from build123d import *

# Parameters (mm, degrees)
F1_DEPTH = 381
F3_DEPTH = 50.8


with BuildPart() as f1:
    # F0 (on Front) → F1 (new body, symmetric)
    with BuildSketch(Plane.XZ):
        with BuildLine():
            ThreePointArc((38.1, 25.4), (34.3802561211, 34.3802561211), (25.4, 38.1))
            Line((25.4, 38.1), (-25.4, 38.1))
            ThreePointArc((-25.4, 38.1), (-34.3802561211, 34.3802561211), (-38.1, 25.4))
            Line((-38.1, 25.4), (-38.1, -25.4))
            ThreePointArc((-38.1, -25.4), (-34.3802561211, -34.3802561211), (-25.4, -38.1))
            Line((-25.4, -38.1), (25.4, -38.1))
            ThreePointArc((25.4, -38.1), (34.3802561211, -34.3802561211), (38.1, -25.4))
            Line((38.1, -25.4), (38.1, 25.4))
        make_face()
        with BuildLine():
            ThreePointArc((25.4, 31.7500010133), (29.890128777, 29.890128777), (31.7500010133, 25.4))
            Line((31.7500010133, 25.4), (31.7500010133, -25.4))
            ThreePointArc((31.7500010133, -25.4), (29.890128777, -29.890128777), (25.4, -31.7500010133))
            Line((25.4, -31.7500010133), (-25.4, -31.7500010133))
            ThreePointArc((-25.4, -31.7500010133), (-29.890128777, -29.890128777), (-31.7500010133, -25.4))
            Line((-31.7500010133, -25.4), (-31.7500010133, 25.4))
            ThreePointArc((-31.7500010133, 25.4), (-29.890128777, 29.890128777), (-25.4, 31.7500010133))
            Line((-25.4, 31.7500010133), (25.4, 31.7500010133))
        make_face(mode=Mode.SUBTRACT)
    extrude(amount=F1_DEPTH, both=True)

    # F2 (on Top) → F3 (cut, symmetric)
    with BuildSketch(Plane.XY):
        Polygon((38.1, -304.8), (-38.1, -381), (38.1, -381), align=None)
        Polygon((38.1, 381), (-38.1, 381), (38.1, 304.8), align=None)
    extrude(amount=F3_DEPTH, both=True, mode=Mode.SUBTRACT)


solid = f1.part
Work out the finished part from the listing and answer in its coordinate system (mm). A direction names the side the tool comes from. Give positions to 0.01 mm unless a question says otherwise; leave off trailing zeros. Write each loop counter-clockwise with the first axis right and the second up, starting at its lowest first coordinate (ties: lowest second). Pieces come first, ordered by that corner, then holes. Notation, with made-up numbers: (43.5, -2.75) - (76.5, -2.75) arc R35 cw to (76.5, 34.25) - close; hole circle Ø4 at (-30.5, 64.25). An arc over 180 degrees is marked (long way). One line per item, written item: value. Start each with the question number.
1. For a pull along Z with two mould halves and no side action, classify faces 3 (the cylindrical face through (34.48, -4.44, 34.28)), 4 (the cylindrical face through (34.28, -4.44, -34.48)), 5 (the flat face through (31.75, -4, 0)) as +Z half, -Z half, draft (parallel to the pull), parting line (faces both ways), or undercut.
2. Find section C-C (y = -79.5). Write down the section's boundary in (x, z), then the cut area to 3 significant figures.
3. Consider probe 1 along Z at (x, y) = (-1, -38.5); probe 2 along Z at (x, y) = (28, 147). Determine where each line is inside the solid, lowest interval first.
4. For faces 1 (the flat face through (-31.75, -5, 0)), 2 (the cylindrical face through (-34.48, -5.33, -34.28)), determine the directions among +Z, -Z, +X, -X, +Y, -Y from which every point of the face is accessible in a straight line to the end or side of a thin tool.
5. Find section A-A (x = -19). Write down the section's boundary in (y, z), then the cut area to 3 significant figures.
6. Find section B-B (z = 2.5). Write down the section's boundary in (x, y).
Geometry results:
1. face 3: +Z half
1. face 4: -Z half
1. face 5: undercut
2. outline: (-38.1, -25.4) arc R12.7 ccw to (-25.4, -38.1) - (25.4, -38.1) arc R12.7 ccw to (38.1, -25.4) - (38.1, 25.4) arc R12.7 ccw to (25.4, 38.1) - (-25.4, 38.1) arc R12.7 ccw to (-38.1, 25.4) - close; hole (-31.75, -25.4) arc R6.35 ccw to (-25.4, -31.75) - (25.4, -31.75) arc R6.35 ccw to (31.75, -25.4) - (31.75, 25.4) arc R6.35 ccw to (25.4, 31.75) - (-25.4, 31.75) arc R6.35 ccw to (-31.75, 25.4) - close
2. area: 1,670 mm2
3. probe 1: -38.1 to -31.75, 31.75 to 38.1
3. probe 2: -37.83 to -31.19, 31.19 to 37.83
4. face 1: +Y, -Y
4. face 2: -Z, -X, +Y, -Y
5. outline: (-361.9, -38.1) - (361.9, -38.1) - (361.9, -31.75) - (-361.9, -31.75) - close; (-361.9, 31.75) - (361.9, 31.75) - (361.9, 38.1) - (-361.9, 38.1) - close
5. area: 9,190 mm2
6. outline: (-38.1, -381) - (-31.75, -374.65) - (-31.75, 374.65) - (-38.1, 381) - close; (31.75, -311.15) - (38.1, -304.8) - (38.1, 304.8) - (31.75, 311.15) - close
